Check sheet for the modelled part. Datum: model origin and axes. Units: mm. Round coordinates to 2 decimals unless told otherwise and drop trailing zeros. Order: outer loops, then holes, each group sorted by start corner. A loop starts at its lowest first (then second) coordinate and runs counter-clockwise, first axis right, second up. Notation, with made-up numbers: (-1.75, 77) -> (8.25, 77) arc R21 cw to (8.25, 106) -> close; hole circle Ø9 at (-14.75, 64.5). An arc over 180 degrees is marked (long way). Use CSV: the item, a comma, the result in double quotes.
```python
from build123d import *

# Parameters (mm, degrees)
SKETCH1_R           = 3.75
BOSS_EXTRUDE1_DEPTH = 1.1
SKETCH2_R           = 1.3
CUT_EXTRUDE1_DEPTH  = 2.1
FILLET1_R           = 0.5


with BuildPart() as part:
    # Sketch1 → Boss-Extrude1 (new body)
    with BuildSketch(Plane(origin=(0, 0, 0), x_dir=(1, 0, 0), z_dir=(0, 1, 0))):
        Circle(SKETCH1_R)
    extrude(amount=BOSS_EXTRUDE1_DEPTH)

    # Sketch2 → Cut-Extrude1 (cut, through all)
    with BuildSketch(Plane(origin=(0, 1.1, 0), x_dir=(1, 0, 0), z_dir=(0, 1, 0))):
        Circle(SKETCH2_R)
    extrude(amount=-CUT_EXTRUDE1_DEPTH, mode=Mode.SUBTRACT)

    # Fillet1
    fillet1_edges = [part.edges().sort_by_distance(p)[0] for p in [
        (-3.75, 0, 0),
        (-3.75, 1.1, 0),
    ]]
    fillet(fillet1_edges, radius=FILLET1_R)


solid = part.part
```
Q1. Scan lines: L1, parallel to Z at x = 0, y = 0.55; L2, parallel to X at y = 0.65, z = -1; L3, parallel to X at y = 0.1, z = -0.75. Record each from-to range of solid material in increasing order.
Result sheet:
L1,"z = -3.75 to -1.3, 1.3 to 3.75"
L2,"x = -3.61 to -0.83, 0.83 to 3.61"
L3,"x = -3.47 to -1.06, 1.06 to 3.47"
Q2. Sectioned sample at B-B, the plane x = 0. Enter the section's corners in (y, z), then the cut area to 3 significant figures.
Result sheet:
outline,"(0, -3.25) arc R0.5 ccw to (0.5, -3.75) -> (0.6, -3.75) arc R0.5 ccw to (1.1, -3.25) -> (1.1, -1.3) -> (0, -1.3) -> close; (0, 1.3) -> (1.1, 1.3) -> (1.1, 3.25) arc R0.5 ccw to (0.6, 3.75) -> (0.5, 3.75) arc R0.5 ccw to (0, 3.25) -> close"
area,"5.18 mm^2"
Q3. Mould release check, pull along X, two halves, no side actions. Record for faces 1 (the face through (1.4, 1.1, 0.7)), 2 (the face through (-0.17, 0.56, -1.29)): pulls with the +X half, pulls with the -X half, needs draft (parallel to the pull), parting line crosses it, or undercut.
Result sheet:
face 1,"needs draft"
face 2,"undercut"
Q4. Sectioned sample at C-C, the plane y = 0.3. Enter the section's corners in (x, z).
Result sheet:
outline,"circle Ø7.42 at (0, 0); hole circle Ø2.6 at (0, 0)"
Q5. Sectioned sample at A-A, the plane z = 0. Enter the section's corners in (x, y), then the cut area to 3 significant figures.
Result sheet:
outline,"(-3.75, 0.5) arc R0.5 ccw to (-3.25, 0) -> (-1.3, 0) -> (-1.3, 1.1) -> (-3.25, 1.1) arc R0.5 ccw to (-3.75, 0.6) -> close; (1.3, 0) -> (3.25, 0) arc R0.5 ccw to (3.75, 0.5) -> (3.75, 0.6) arc R0.5 ccw to (3.25, 1.1) -> (1.3, 1.1) -> close"
area,"5.18 mm^2"
